```python
from build123d import *

# Parameters (mm, degrees)
SKETCH_1_R      = 2.11
SKETCH_1_R_2    = 1.25
EXTRUDE_1_DEPTH = 1.6
FILLET_1_R      = 2


with BuildPart() as part:
    # 草图1 → 凸台-拉伸1 (new body)
    with BuildSketch(Plane.XY):
        Polygon((12, 0), (0, 0), (0, -24), (12, -24), (12, -21), (24, -21), (24, -3), (12, -3), align=None)
        with Locations((13, -7)):
            Circle(SKETCH_1_R, mode=Mode.SUBTRACT)
        with Locations((13, -17)):
            Circle(SKETCH_1_R, mode=Mode.SUBTRACT)
        with Locations((3, -17)):
            Circle(SKETCH_1_R, mode=Mode.SUBTRACT)
        with Locations((8, -17)):
            Circle(SKETCH_1_R_2, mode=Mode.SUBTRACT)
        with Locations((3, -7)):
            Circle(SKETCH_1_R, mode=Mode.SUBTRACT)
        with Locations((8, -7)):
            Circle(SKETCH_1_R_2, mode=Mode.SUBTRACT)
    extrude(amount=EXTRUDE_1_DEPTH)

    # 圆角1
    fillet_1_edges = [part.edges().sort_by_distance(p)[0] for p in [
        (12, -24, 0.8),
        (0, -24, 0.8),
        (0, 0, 0.8),
        (12, 0, 0.8),
        (24, -3, 0.8),
        (24, -21, 0.8),
    ]]
    fillet(fillet_1_edges, radius=FILLET_1_R)


solid = part.part
```
The listing builds one solid part. Answer for the finished solid, in the listing's coordinates (mm). A direction names the side the tool comes from. Give positions to 0.01 mm unless a question says otherwise; leave off trailing zeros. Order: outer loops, then holes, each group sorted by start corner. A loop starts at its lowest first (then second) coordinate and runs counter-clockwise, first axis right, second up.
Item 1: For a pull along X with two mould halves and no side action, classify faces 4 (the face through (12, -12, 1.6)), 5 (the face through (4.1, -5.2, 0.8)), 6 (the face through (0.57, -23.4, 0.81)), 7 (the face through (11.4, -23.43, 0.81)) as pulls with the +X half, pulls with the -X half, needs draft (parallel to the pull), parting line crosses it, or undercut.
From the geometry:
face 4: needs draft
face 5: undercut
face 6: pulls with the -X half
face 7: pulls with the +X half
Item 2: Given pin 1 Ø8 at (x, y) = (21.5, -20.5) entering from -Z; pin 2 Ø2 at (x, y) = (8, -17) entering from -Z; pin 3 Ø0.5 at (x, z) = (16, 1) entering from -Y, each flat-ended and moving along its own axis, determine where each tip first touches the part or whether it passes through.
From the geometry:
pin 1: stops at z = 0
pin 2: passes through
pin 3: stops at y = -21
Item 3: The part is cut by section D-D, the plane x = 3. Give the vertices of the cut face in (y, z), and give its area (3 significant figures).
From the geometry:
outline: (-24, 0) - (-19.11, 0) - (-19.11, 1.6) - (-24, 1.6) - close; (-14.89, 0) - (-9.11, 0) - (-9.11, 1.6) - (-14.89, 1.6) - close; (-4.89, 0) - (0, 0) - (0, 1.6) - (-4.89, 1.6) - close
area: 24.9 mm2
Item 4: Which of the six approach directions +Z, -Z, +X, -X, +Y, -Y give full straight-line access (tool end or side, diameter ignored) to faces 1 (the face through (17, -21, 1)), 2 (the face through (12, -2.5, 0.8)), 3 (the face through (11.445, -5.574, 0.789))?
From the geometry:
face 1: +Z, -Z, +X, -Y
face 2: +Z, -Z, +X, +Y
face 3: +Z, -Z
Item 5: Find the intervals of material crossed by probe 1 along Y at (x, z) = (3, 0.5); probe 2 along Y at (x, z) = (13, 0.65); probe 3 along X at (y, z) = (-17.5, 0.75), in increasing order.
From the geometry:
probe 1: y = -24 to -19.11, -14.89 to -9.11, -4.89 to 0
probe 2: y = -21 to -19.11, -14.89 to -9.11, -4.89 to -3
probe 3: x = 0 to 0.95, 5.05 to 6.85, 9.15 to 10.95, 15.05 to 24
Item 6: The part is cut by section B-B, the plane y = -7. Give the vertices of the cut face in (x, z), and give its area (3 significant figures).
From the geometry:
outline: (0, 0) - (0.89, 0) - (0.89, 1.6) - (0, 1.6) - close; (5.11, 0) - (6.75, 0) - (6.75, 1.6) - (5.11, 1.6) - close; (9.25, 0) - (10.89, 0) - (10.89, 1.6) - (9.25, 1.6) - close; (15.11, 0) - (24, 0) - (24, 1.6) - (15.11, 1.6) - close
area: 20.9 mm2
Item 7: The part is cut by section A-A, the plane x = 8.75. Give the vertices of the cut face in (y, z).
From the geometry:
outline: (-24, 0) - (-18, 0) - (-18, 1.6) - (-24, 1.6) - close; (-16, 0) - (-8, 0) - (-8, 1.6) - (-16, 1.6) - close; (-6, 0) - (0, 0) - (0, 1.6) - (-6, 1.6) - close
Item 8: The part is cut by section C-C, the plane z = 0.45. Give the vertices of the cut face in (x, y).
From the geometry:
outline: (0, -22) arc R2 ccw to (2, -24) - (10, -24) arc R2 ccw to (12, -22) - (12, -21) - (22, -21) arc R2 ccw to (24, -19) - (24, -5) arc R2 ccw to (22, -3) - (12, -3) - (12, -2) arc R2 ccw to (10, 0) - (2, 0) arc R2 ccw to (0, -2) - close; hole circle Ø4.22 at (3, -17); hole circle Ø4.22 at (3, -7); hole circle Ø2.5 at (8, -17); hole circle Ø2.5 at (8, -7); hole circle Ø4.22 at (13, -17); hole circle Ø4.22 at (13, -7)
